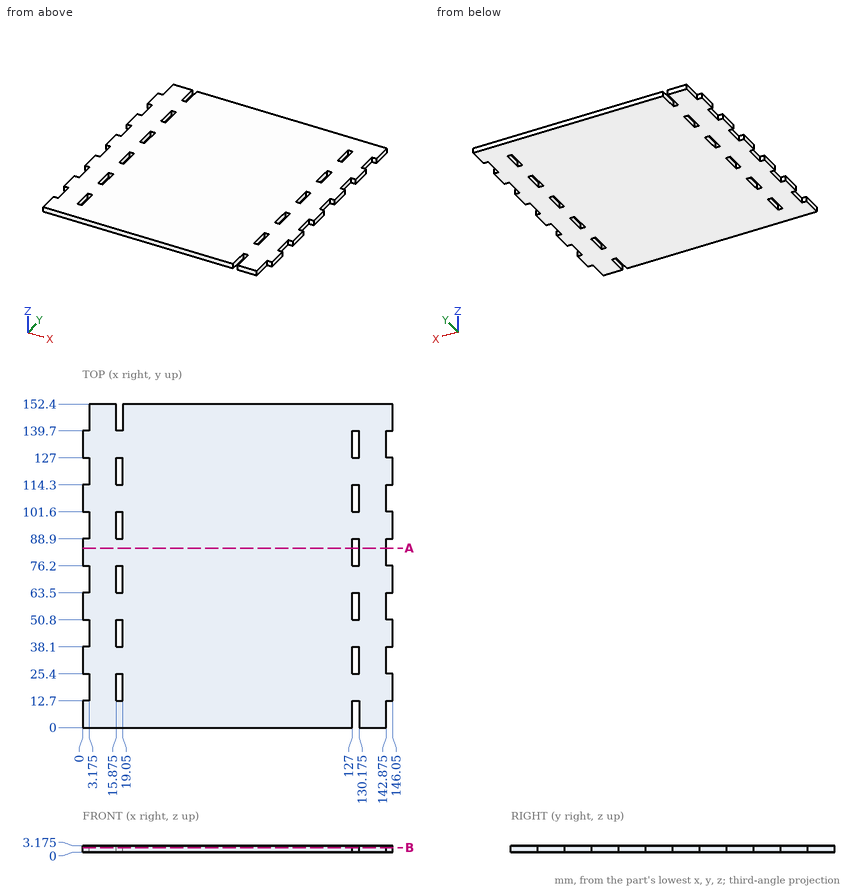
Input: dimensioned drawing with shaded views. Units: mm. Origin: part minimum x, y, z. Give positions to 0.01 mm unless a question says otherwise; leave off trailing zeros. Loops run counter-clockwise (first coordinate to the right, second up) from the corner with the lowest first, then second, coordinate; pieces in that order, holes last. Notation, with made-up numbers: (69.25, -36.5) - (116.25, -36.5) arc R19 ccw to (116.25, 0.5) - close; hole circle Ø2 at (-5.75, 51). An arc over 180 degrees is marked (long way). Answer as CSV lines item,"result". Start each with the question number.
(1) Section query A-A (y = 84.5). Output: boundary loops of the cut face in (x, z) (3 decimals), and give its area (3 significant figures).
(2) Section query B-B (z = 2.3). Give the number of separate pieces and of enclosed holes in the cut face, and give its area (3 significant figures).
(3) Ray query, line 1 along X through (y, z) = (50, 2.7) (3 decimals); line 2 along X through (y, z) = (139, 0.95) (3 decimals). Return the intervals inside material, ascending. Write a range as [from, to].
(4) Pin query (flat end, axial travel): P1, Ø1, axis at y = 31.5, z = 1.5, coming from the +X side (3 decimals); P2, Ø1, axis at y = 72, z = 1.5, coming from the -X side (3 decimals). Return the tip coordinate at first contact, or that it passes through.
Worked answers:
1,outline,"(0, 0) - (127, 0) - (127, 3.175) - (0, 3.175) - close; (130.175, 0) - (142.875, 0) - (142.875, 3.175) - (130.175, 3.175) - close"
1,area,"444 mm^2"
2,separate pieces,"1"
2,enclosed holes,"10"
2,area,"21,300 mm^2"
3,line 1,"x = [3.175, 15.875], [19.05, 146.05]"
3,line 2,"x = [0, 127], [130.175, 142.875]"
4,P1,"stops at x = 142.875"
4,P2,"stops at x = 3.175"
